```python
from build123d import *

# Parameters (mm, degrees)
BOSS_EXTRUDE1_DEPTH = 25
SHELL1_T            = -3


with BuildPart() as part:
    # Sketch1 → Boss-Extrude1 (new body)
    with BuildSketch(Plane(origin=(0, 0, 0), x_dir=(1, 0, 0), z_dir=(0, 1, 0))):
        Polygon((-174.5, 170.560948081), (174.5, 170.560948081), (174.5, 195.560948081), (-199.5, 195.560948081), align=None)
    extrude(amount=BOSS_EXTRUDE1_DEPTH)

    # Shell1
    shell1_openings = [part.faces().sort_by_distance(p)[0] for p in [
        (174.5, 12.5, -183.060948081),
        (-187, 12.5, -183.060948081),
    ]]
    offset(amount=SHELL1_T, openings=shell1_openings, kind=Kind.INTERSECTION)


solid = part.part
```
For this review, take the finished solid that the model builds, in its own axes (mm). A direction names the side the tool comes from. Round coordinates to 2 decimals unless told otherwise and drop trailing zeros. Write each loop counter-clockwise with the first axis right and the second up, starting at its lowest first coordinate (ties: lowest second). Pieces come first, ordered by that corner, then holes. Notation, with made-up numbers: (45.25, 61.5) - (64.25, 61.5) arc R35 ccw to (64.25, 96.5) - close; hole circle Ø4 at (-6, -12.5). An arc over 180 degrees is marked (long way). Use CSV: the item, a comma, the result in double quotes.
1) Add section C-C on z = -185. Write out the cut boundary in (x, y).
Conclusion:
outline,"(-188.94, 0) - (174.5, 0) - (174.5, 3) - (-188.94, 3) - close; (-188.94, 22) - (174.5, 22) - (174.5, 25) - (-188.94, 25) - close"
2) Add section A-A on y = 8.75. Write out the cut boundary in (x, z).
Conclusion:
outline,"(-199.5, -195.56) - (174.5, -195.56) - (174.5, -192.56) - (-196.5, -192.56) - close; (-177.5, -173.56) - (174.5, -173.56) - (174.5, -170.56) - (-174.5, -170.56) - close"
3) The part is to be moulded in two halves that separate along Y. For faces 1 (the flat face through (-2, 12, -170.561)), 2 (the flat face through (-8, 12, -192.561)), 3 (the flat face through (-15, 0, -183)), say which applies: pulls with the +Y half, pulls with the -Y half, needs draft (parallel to the pull), parting line crosses it, or undercut.
Conclusion:
face 1,"needs draft"
face 2,"undercut"
face 3,"pulls with the -Y half"
4) Clearance check with a flat-ended pin moving along its axis: pin 1 Ø2 at (y, z) = (8.5, -190.5) entering from -X. State where the tip first meets the part, or that it passes through.
Conclusion:
pin 1,"passes through"
5) Add section B-B on x = -99. Write out the cut boundary in (y, z), and give its area (3 significant figures).
Conclusion:
outline,"(0, -195.56) - (25, -195.56) - (25, -170.56) - (0, -170.56) - close; hole (3, -192.56) - (22, -192.56) - (22, -173.56) - (3, -173.56) - close"
area,"264 mm^2"
6) For faces 4 (the flat face through (-15, 25, -183)), 5 (the flat face through (-14, 22, -183)), list the 3-axis set-ups (+Z, -Z, +X, -X, +Y, -Y) from which the entire face can be reached by the end or side of a thin tool; tool diameter is ignored.
Conclusion:
face 4,"+Z, -Z, +X, -X, +Y"
face 5,"+X, -X"
7) Wall thickness on line 1 along Y through (x, z) = (93, -175.5); line 2 along Z through (x, y) = (-144.5, 7.5); line 3 along X through (y, z) = (14, -171.5): over which ranges is each line inside the solid? List them lowest first. Write a range as from..to.
Conclusion:
line 1,"y = 0..3, 22..25"
line 2,"z = -195.56..-192.56, -173.56..-170.56"
line 3,"x = -175.44..174.5"
